```python
from build123d import *

# Parameters (mm, degrees)
SKETCH2_R           = 4.05
BOSS_EXTRUDE1_DEPTH = 12.5
FILLET1_R           = 2
CUT_EXTRUDE1_DEPTH  = 61.03151231
BOSS_EXTRUDE2_START = -12.5
BOSS_EXTRUDE2_DEPTH = 12.5
FILLET2_R           = 1
SKETCH7_R           = 1.45
CUT_EXTRUDE2_DEPTH  = 61.585751092


with BuildPart() as part:
    # Sketch2 → Boss-Extrude1 (new body)
    with BuildSketch(Plane(origin=(0, 0, 0), x_dir=(1, 0, 0), z_dir=(0, 1, 0))):
        with BuildLine():
            Line((-10, 0), (0, -70))
            Line((0, -70), (10, 0))
            ThreePointArc((10, 0), (0, 10), (-10, 0))
        make_face()
        with Locations(Location((0, 3.5, 0), (0, 0, 270))):
            Circle(SKETCH2_R, mode=Mode.SUBTRACT)
    extrude(amount=BOSS_EXTRUDE1_DEPTH)

    # Fillet1
    fillet1_edges = [part.edges().sort_by_distance(p)[0] for p in [
        (0, 6.25, 70),
    ]]
    fillet(fillet1_edges, radius=FILLET1_R)

    # Sketch5 → Cut-Extrude1 (cut, through all)
    with BuildSketch(Plane(origin=(0, 12.5, 0), x_dir=(1, 0, 0), z_dir=(0, 1, 0))):
        with BuildLine():
            Line((-1.371121558, 3.757662262), (-1.371121558, 13.050926013))
            Line((-1.371121558, 13.050926013), (1.374099614, 13.050926013))
            Line((1.374099614, 13.050926013), (1.374099614, 3.756574271))
            ThreePointArc((1.374099614, 3.756574271), (0.697747417, 3.938673449), (0, 4))
            ThreePointArc((0, 4), (-0.69618638, 3.938949673), (-1.371121558, 3.757662262))
        make_face()
    extrude(amount=-CUT_EXTRUDE1_DEPTH, mode=Mode.SUBTRACT)

    # Sketch6 → Boss-Extrude2 (add)
    with BuildSketch(Plane(origin=(0, 12.5, 0), x_dir=(1, 0, 0), z_dir=(0, 1, 0)).offset(BOSS_EXTRUDE2_START)):
        with BuildLine():
            Line((-2.91788587, 9.564828386), (-2.91788587, 15.613591417))
            Line((-2.91788587, 15.613591417), (-1.371121558, 15.613591417))
            Line((-1.371121558, 15.613591417), (-1.371121558, 9.905555294))
            ThreePointArc((-1.371121558, 9.905555294), (-2.151260069, 9.765862999), (-2.91788587, 9.564828386))
        make_face()
        with BuildLine():
            Line((1.374099614, 9.905142616), (1.374099614, 15.613591417))
            Line((1.374099614, 15.613591417), (2.917072625, 15.613591417))
            Line((2.917072625, 15.613591417), (2.917072625, 9.56507644))
            ThreePointArc((2.917072625, 9.56507644), (2.152312953, 9.765631006), (1.374099614, 9.905142616))
        make_face()
    extrude(amount=BOSS_EXTRUDE2_DEPTH)

    # Fillet2
    fillet2_edges = [part.edges().sort_by_distance(p)[0] for p in [
        (-2.91788587, 6.25, -15.613591417),
        (2.917072625, 6.25, -15.613591417),
    ]]
    fillet(fillet2_edges, radius=FILLET2_R)

    # Sketch7 → Cut-Extrude2 (cut, through all)
    with BuildSketch(Plane(origin=(2.917072625, 0, 0), x_dir=(0, 0, -1), z_dir=(1, 0, 0))):
        with Locations((12.36507644, 6.25)):
            Circle(SKETCH7_R)
    extrude(amount=-CUT_EXTRUDE2_DEPTH, mode=Mode.SUBTRACT)


solid = part.part
```
CAD build for the part. Positions are in the model's coordinates, mm. A direction names the side the tool comes from. Coordinates: 2 decimals unless noted, no trailing zeros. Write each loop counter-clockwise with the first axis right and the second up, starting at its lowest first coordinate (ties: lowest second). Pieces come first, ordered by that corner, then holes. Notation, with made-up numbers: (87.5, 33.5) -> (120.5, 33.5) arc R27 ccw to (120.5, 72.5) -> close; hole circle Ø3 at (-9.5, 65.25). An arc over 180 degrees is marked (long way). Return JSON: item names as keys, results as strings. Group by question number.
Q1. Cut at A-A, the plane y = 6.25. Give the cut face in (x, z).
Q2. Cut at B-B, the plane z = -3.5. Give the cut face in (x, y).
Q3. Drill centre lines: line 1 (X direction, y = 1.25, z = -10.5); line 2 (X direction, y = 7.25, z = -7.5); line 3 (X direction, y = 10.5, z = 5.5). Where is each one in solid material? Low to high.
Q4. Which spindle directions (+Z, -Z, +X, -X, +Y, -Y) get a long thin tool onto all of the face, cutting with end or side? Do faces 4 (the face through (2.917, 4.8, -11.6)), 5 (the face through (-1.371, 6.2, -10.6)), 6 (the face through (-2.918, 5, -11)), 7 (the face through (-0.04, 6.338, 57.857)). Say none if no direction does.
Q5. Cut at D-D, the plane z = 49. Give the cut face in (x, y).
Q6. Flat gauge pins, fed straight in: pin 1 (5.5 mm diameter, centred on y = 8.5, z = -11, fed in from +X); pin 2 (2 mm diameter, centred on x = 7.5, y = 11, fed in from -Z); pin 3 (5.5 mm diameter, centred on y = 4, z = -13, fed in from -X); pin 4 (2.5 mm diameter, centred on y = 6.25, z = -12.37, fed in from +X). Where does each tip first touch, or does it go through?
Q7. Pull direction Z, two halves, no side cores. Call faces 1 (the face through (8, 6, -6)), 2 (the face through (6, 6, 28)), 3 (the face through (-0.16, 6.162, 0.547)): released by +Z, released by -Z, zero draft, split by the parting line, or undercut.
Q8. Cut at C-C, the plane y = 3. Give the cut face in (x, z), then the cut area to 3 significant figures.
Returned:
{
 "1": {"outline": "(-10, 0) arc R10 ccw to (-2.92, -9.56) -> (-2.92, -10.92) -> (-1.37, -10.92) -> (-1.37, -7.31) arc R4.05 cw (long way) to (1.37, -7.31) -> (1.37, -10.92) -> (2.92, -10.92) -> (2.92, -9.57) arc R10 ccw to (10, 0) -> (1.98, 56.14) arc R2 ccw to (-1.98, 56.14) -> close; (-2.92, -14.61) arc R1 ccw to (-1.92, -15.61) -> (-1.37, -15.61) -> (-1.37, -13.82) -> (-2.92, -13.82) -> close; (1.37, -15.61) -> (1.92, -15.61) arc R1 ccw to (2.92, -14.61) -> (2.92, -13.82) -> (1.37, -13.82) -> close"},
 "2": {"outline": "(-9.37, 0) -> (-4.05, 0) -> (-4.05, 12.5) -> (-9.37, 12.5) -> close; (4.05, 0) -> (9.37, 0) -> (9.37, 12.5) -> (4.05, 12.5) -> close"},
 "3": {"line 1": "x = -2.92 to -1.37, 1.37 to 2.92", "line 2": "x = -6.61 to -1.37, 1.37 to 6.61", "line 3": "x = -9.21 to 9.21"},
 "4": {"face 4": "-Z, +X, +Y, -Y", "face 5": "-Z, +Y, -Y", "face 6": "-Z, -X, +Y, -Y", "face 7": "+Z, +Y, -Y"},
 "5": {"outline": "(-3, 0) -> (3, 0) -> (3, 12.5) -> (-3, 12.5) -> close"},
 "6": {"pin 1": "stops at x = 5.65", "pin 2": "stops at z = -7.6", "pin 3": "stops at x = -2.92", "pin 4": "passes through"},
 "7": {"face 1": "released by -Z", "face 2": "released by +Z", "face 3": "undercut"},
 "8": {"outline": "(-10, 0) arc R10 ccw to (-2.92, -9.56) -> (-2.92, -14.61) arc R1 ccw to (-1.92, -15.61) -> (-1.37, -15.61) -> (-1.37, -7.31) arc R4.05 cw (long way) to (1.37, -7.31) -> (1.37, -15.61) -> (1.92, -15.61) arc R1 ccw to (2.92, -14.61) -> (2.92, -9.57) arc R10 ccw to (10, 0) -> (1.98, 56.14) arc R2 ccw to (-1.98, 56.14) -> close", "area": "794 mm2"}
}
